from build123d import *

# Parameters (mm, degrees)
SKETCH_1_W               = 23
SKETCH_1_H               = 17
SKETCH_1_R               = 1.1
EXTRUDE_1_DEPTH          = 3
EXTRUDE_2_DEPTH          = 6
CUT_EXTRUDE_1_DEPTH      = 23.349496639
CUT_EXTRUDE_1_DEPTH_BACK = 1
SKETCH_3_R               = 2.25
CUT_EXTRUDE_2_REACH      = 24.349
SKETCH_4_W               = 4.5
SKETCH_4_H               = 17
CUT_EXTRUDE_3_DEPTH      = 2
SKETCH_6_R               = 2.15
CUT_EXTRUDE_4_DEPTH      = 4
SKETCH_7_W               = 16.5
SKETCH_7_H               = 10
EXTRUDE_3_DEPTH          = 4
SKETCH_8_R               = 2.15
CUT_EXTRUDE_5_DEPTH      = 4
CHAMFER_1_SIZE           = 1
CHAMFER_1_SIZE2          = 1.732050808
CHAMFER_2_SIZE           = 4
CUT_EXTRUDE_6_DEPTH      = 1
FILLET_1_R               = 2
CUT_EXTRUDE_7_REACH      = 21.881
FILLET_2_R               = 1
CHAMFER_3_SIZE           = 2
CHAMFER_3_SIZE2          = 2.813680863


with BuildPart() as part:
    # 草图1 → 凸台-拉伸1 (new body)
    with BuildSketch(Plane.XY):
        with Locations((4, 6)):
            Rectangle(SKETCH_1_W, SKETCH_1_H)
        Circle(SKETCH_1_R, mode=Mode.SUBTRACT)
        with Locations((8, 0)):
            Circle(SKETCH_1_R, mode=Mode.SUBTRACT)
        with Locations((0, 12)):
            Circle(SKETCH_1_R, mode=Mode.SUBTRACT)
        with Locations((8, 12)):
            Circle(SKETCH_1_R, mode=Mode.SUBTRACT)
    extrude(amount=EXTRUDE_1_DEPTH)

    # 草图2 → 凸台-拉伸2 (add)
    with BuildSketch(Plane.ZY.offset(7.5)):
        Polygon((5.5, 14.5), (10, -2.5), (5.5, -2.5), (0, -2.5), (0, 14.5), align=None)
    extrude(amount=-EXTRUDE_2_DEPTH)

    # 草图3 → 切除-拉伸1 (cut, two sides: drawn at the far end of the back side and taken through both)
    with BuildSketch(Plane.XY.offset(3).offset(-CUT_EXTRUDE_1_DEPTH_BACK)):
        with Locations(Location((0, 12, 0), (0, 0, 228.189685104))):
            Circle(SKETCH_3_R)
        with Locations((8, 12)):
            Circle(SKETCH_3_R)
        with Locations(Location((0, 0, 0), (0, 0, 131.810314896))):
            Circle(SKETCH_3_R)
        with Locations((8, 0)):
            Circle(SKETCH_3_R)
    extrude(amount=CUT_EXTRUDE_1_DEPTH + CUT_EXTRUDE_1_DEPTH_BACK, mode=Mode.SUBTRACT)

    # 草图4 → 切除-拉伸2 (cut, up to next)
    with BuildSketch(Plane.XY.offset(3), mode=Mode.PRIVATE) as cut_extrude_2_sk1:
        with Locations((13.25, 6)):
            Rectangle(SKETCH_4_W, SKETCH_4_H)
    cut_extrude_2_tool1 = extrude(cut_extrude_2_sk1.sketch, amount=-CUT_EXTRUDE_2_REACH, mode=Mode.PRIVATE) & part.part
    add(cut_extrude_2_tool1.solids().sort_by_distance((13.25, 6, 3))[0], mode=Mode.SUBTRACT)

    # 草图5 → 切除-拉伸3 (cut)
    with BuildSketch(Plane.ZY.offset(7.5)):
        Polygon((0, 14.5), (0, -2.5), (10, -2.5), (5.5, 14.5), align=None)
    extrude(amount=-CUT_EXTRUDE_3_DEPTH, mode=Mode.SUBTRACT)

    # 草图6 → 切除-拉伸4 (cut)
    with BuildSketch(Plane.ZY.offset(5.5)):
        with Locations(Location((3.875, 6, 0), (0, 0, 270))):
            Circle(SKETCH_6_R)
    extrude(amount=-CUT_EXTRUDE_4_DEPTH, mode=Mode.SUBTRACT)

    # 草图7 → 凸台-拉伸3 (add)
    with BuildSketch(Plane.XZ.offset(2.5)):
        with Locations((2.75, 5)):
            Rectangle(SKETCH_7_W, SKETCH_7_H)
    extrude(amount=EXTRUDE_3_DEPTH)

    # 草图8 → 切除-拉伸5 (cut)
    with BuildSketch(Plane.XZ.offset(6.5)):
        with Locations(Location((1.5, 5.7, 0), (0, 0, 270))):
            Circle(SKETCH_8_R)
    extrude(amount=-CUT_EXTRUDE_5_DEPTH, mode=Mode.SUBTRACT)

    # 倒角1
    chamfer_1_edges = [part.edges().sort_by_distance(p)[0] for p in [
        (2.75, -6.5, 0),
    ]]
    chamfer_1_side = [part.faces().sort_by_distance(p)[0] for p in [
        (2.692629218, 3.908206749, 0),
    ]]
    chamfer(chamfer_1_edges, length=CHAMFER_1_SIZE, length2=CHAMFER_1_SIZE2, reference=chamfer_1_side[0])

    # 倒角2
    chamfer_2_edges = [part.edges().sort_by_distance(p)[0] for p in [
        (11, -4.5, 10),
    ]]
    chamfer(chamfer_2_edges, length=CHAMFER_2_SIZE)

    # 草图9 → 切除-拉伸6 (cut)
    with BuildSketch(Plane.XY.offset(3)):
        with BuildLine():
            Line((-1.5, 13.677050983), (-1.5, 14.5))
            Line((-1.5, 14.5), (2.25, 14.5))
            Line((2.25, 14.5), (2.25, 12))
            ThreePointArc((2.25, 12), (0.918558654, 14.053959591), (-1.5, 13.677050983))
        make_face()
        with BuildLine():
            Line((5.75, 12), (5.75, 14.5))
            Line((5.75, 14.5), (11, 14.5))
            Line((11, 14.5), (11, 9.75))
            Line((11, 9.75), (8, 9.75))
            ThreePointArc((8, 9.75), (9.590990258, 13.590990258), (5.75, 12))
        make_face()
        with BuildLine():
            Line((2.25, 0), (2.25, -2.5))
            Line((2.25, -2.5), (-1.5, -2.5))
            Line((-1.5, -2.5), (-1.5, -1.677050983))
            ThreePointArc((-1.5, -1.677050983), (0.918558654, -2.053959591), (2.25, 0))
        make_face()
        with BuildLine():
            Line((5.75, 0), (5.75, -2.5))
            Line((5.75, -2.5), (11, -2.5))
            Line((11, -2.5), (11, 2.25))
            Line((11, 2.25), (8, 2.25))
            ThreePointArc((8, 2.25), (9.590990258, -1.590990258), (5.75, 0))
        make_face()
    extrude(amount=-CUT_EXTRUDE_6_DEPTH, mode=Mode.SUBTRACT)

    # 圆角1
    fillet_1_edges = [part.edges().sort_by_distance(p)[0] for p in [
        (11, 14.5, 1),
    ]]
    fillet(fillet_1_edges, radius=FILLET_1_R)

    # 草图10 → 切除-拉伸7 (cut, up to next)
    with BuildSketch(Plane.XY.offset(2), mode=Mode.PRIVATE) as cut_extrude_7_sk1:
        with BuildLine():
            Line((4, 14.5), (11, 14.5))
            Line((11, 14.5), (11, 6))
            Line((11, 6), (4, 6))
            Line((4, 6), (4, 9.75))
            Line((4, 9.75), (0, 9.75))
            ThreePointArc((0, 9.75), (1.590990258, 10.409009742), (2.25, 12))
            Line((2.25, 12), (2.25, 14.5))
            Line((2.25, 14.5), (4, 14.5))
        make_face()
    cut_extrude_7_tool1 = extrude(cut_extrude_7_sk1.sketch, amount=CUT_EXTRUDE_7_REACH, mode=Mode.PRIVATE) & part.part
    add(cut_extrude_7_tool1.solids().sort_by_distance((6.881457, 10.476255, 2))[0], mode=Mode.SUBTRACT)

    # 圆角2
    fillet_2_edges = [part.edges().sort_by_distance(p)[0] for p in [
        (4, 9.75, 2.5),
        (4, 6, 2.5),
    ]]
    fillet(fillet_2_edges, radius=FILLET_2_R)

    # 倒角3
    chamfer_3_edges = [part.edges().sort_by_distance(p)[0] for p in [
        (-3.5, 14.5, 5.5),
    ]]
    chamfer_3_side = [part.faces().sort_by_distance(p)[0] for p in [
        (0.040697674, 14.5, 1.895348837),
    ]]
    chamfer(chamfer_3_edges, length=CHAMFER_3_SIZE, length2=CHAMFER_3_SIZE2, reference=chamfer_3_side[0])


solid = part.part
Read the model definition and answer for the solid it produces. Units are mm, in the model's axes. A direction names the side the tool comes from. Give positions to 0.01 mm unless a question says otherwise; leave off trailing zeros. Write each loop counter-clockwise with the first axis right and the second up, starting at its lowest first coordinate (ties: lowest second). Pieces come first, ordered by that corner, then holes. Notation, with made-up numbers: (-25, 43.25) - (12, 43.25) arc R25 cw to (12, 67.25) - close; hole circle Ø7 at (28.25, 3). An arc over 180 degrees is marked (long way). Answer in a Markdown table with one row per item. Add a question column.
Item 1: Section B-B, the plane x = -3.75 is taken. Write down the section's boundary in (y, z) (3 decimals), and give its area (3 significant figures).
Item 2: Find the intervals of material crossed by L1, parallel to X at y = 0, z = 0.55; L2, parallel to Y at x = 8, z = 1.3; L3, parallel to Z at x = -0.25, y = -1.5, in increasing order.
Item 3: Section D-D, the plane y = 5.25 is taken. Write down the section's boundary in (x, z), and give its area (3 significant figures).
Item 4: A tool of negligible diameter and unlimited length cuts with its end or side. For faces 1 (the face through (3, 5, 0)), 2 (the face through (1.5, 9.75, 2.5)), 3 (the face through (6.43, 1.61, 2.49)), from which of +Z, -Z, +X, -X, +Y, -Y can it reach the whole face along a straight path? Write none if from no direction.
Item 5: Section C-C, the plane z = 5.7 is taken. Write down the section's boundary in (x, y), and give its area (3 significant figures).
Item 6: Section A-A, the plane y = 11.5 is taken. Write down the section's boundary in (x, z), and give its area (3 significant figures).
Item 7: Determine the mould class of faces 4 (the face through (-3.528, 4.74, 8.084)), 5 (the face through (-1.5, 5, 6)), 6 (the face through (9.016, -0.421, 0.986)) for opening direction X: pulls with the +X half, pulls with the -X half, needs draft (parallel to the pull), parting line crosses it, or undercut.
Item 8: Flat-ended cylindrical pins translate along their axes: P1, Ø1, axis at x = 4.5, z = 5, coming from the +Y side; P2, Ø4.5, axis at y = 4, z = 6.5, coming from the +X side; P3, Ø6, axis at x = 6, y = 1.5, coming from the +Z side. Find the tip coordinate at first contact, or state that the pin passes through.
Recorded:
| question | item | result |
|---|---|---|
| 1 | outline | (-6.5, 1.732) - (-5.5, 0) - (14.5, 0) - (14.5, 3.5) - (11.78, 6.22) - (-2.5, 10) - (-6.5, 10) - close; hole circle Ø4.3 at (6, 3.875) |
| 1 | area | 154 mm2 |
| 2 | L1 | x = -5.5 to -1.1, 1.1 to 6.9, 9.1 to 11 |
| 2 | L2 | y = -6.25 to -1.1, 1.1 to 10.9, 13.1 to 14.5 |
| 2 | L3 | z = 0 to 2 |
| 3 | outline | (-5.5, 0) - (11, 0) - (11, 3) - (-1.5, 3) - (-1.5, 1.86) - (-5.5, 1.86) - close; (-5.5, 5.89) - (-1.5, 5.89) - (-1.5, 7.95) - (-5.5, 7.95) - close |
| 3 | area | 53.2 mm2 |
| 4 | face 1 | -Z, +X, -X, +Y, -Y |
| 4 | face 2 | +Z, +X, +Y |
| 4 | face 3 | +Z, +X |
| 5 | outline | (-5.5, -6.5) - (-0.65, -6.5) - (-0.65, -2.5) - (-1.5, -2.5) - (-1.5, -1.68) arc R2.25 cw to (-1.5, 1.68) - (-1.5, 4.86) - (-5.5, 4.86) - close; (-5.5, 7.14) - (-1.5, 7.14) - (-1.5, 10.32) arc R2.25 cw to (-2.23, 12.3) - (-5.5, 12.3) - close; (3.65, -6.5) - (11, -6.5) - (11, -2.5) - (3.65, -2.5) - close |
| 5 | area | 96.1 mm2 |
| 6 | outline | (-5.5, 0) - (-0.98, 0) - (-0.98, 2) - (-2.19, 2) - (-2.19, 6.29) - (-5.5, 6.29) - close; (0.98, 0) - (7.02, 0) - (7.02, 2) - (0.98, 2) - close; (8.98, 0) - (11, 0) - (11, 2) - (8.98, 2) - close |
| 6 | area | 39.4 mm2 |
| 7 | face 4 | needs draft |
| 7 | face 5 | pulls with the +X half |
| 7 | face 6 | undercut |
| 8 | P1 | stops at y = -2.5 |
| 8 | P2 | stops at x = -1.5 |
| 8 | P3 | stops at z = 3 |
